from build123d import *

# Parameters (mm, degrees)
SKETCH_1_W          = 18
SKETCH_1_H          = 49
EXTRUDE_1_DEPTH     = 2
CUT_EXTRUDE_1_DEPTH = 0.1


with BuildPart() as part:
    # ｽｹｯﾁ1 → ﾎﾞｽ - 押し出し1 (new body)
    with BuildSketch(Plane.XY):
        with Locations((9, 24.5)):
            Rectangle(SKETCH_1_W, SKETCH_1_H)
    extrude(amount=EXTRUDE_1_DEPTH)

    # ｽｹｯﾁ2 → ｶｯﾄ - 押し出し1 (cut)
    with BuildSketch(Plane.XY.offset(2)):
        with BuildLine():
            add(Edge.make_bspline(
                [(0.915865385, 24.396709736), (0.91809708, 24.77837232), (0.922432179, 25.519757391), (0.970658757, 26.600060045), (1.05077314, 27.613522012), (1.160564909, 28.5601918), (1.29417331, 29.440313805), (1.472532246, 30.251535992), (1.675365778, 30.997612959), (1.910445811, 31.68097761), (2.175702018, 32.310836625), (2.464406542, 32.898836655), (2.788017018, 33.444088016), (3.128038515, 33.95529334), (3.498234931, 34.42408455), (3.888071345, 34.85708195), (4.312763039, 35.244278306), (4.757873149, 35.597018327), (5.227431594, 35.906237054), (5.708054019, 36.178602651), (6.203048578, 36.411283891), (6.713766716, 36.594234892), (7.235618047, 36.745347974), (7.77042684, 36.848687065), (8.31907612, 36.913708174), (8.689404274, 36.919924378), (8.877216046, 36.923076923)],
                knots=[0, 0, 0, 0, 1.646270934, 3.197905019, 4.663502075, 6.030701355, 7.308322542, 8.50163776, 9.611534131, 10.641858119, 11.616356847, 12.558055219, 13.465016945, 14.349605745, 15.204443733, 16.039544428, 16.859896111, 17.680448484, 18.487036065, 19.28249412, 20.06191084, 20.843045899, 21.620316918, 22.403196591, 23.190181807, 24, 24, 24, 24], degree=3))
            add(Edge.make_bspline(
                [(8.877216046, 36.923076923), (9.066596712, 36.919758038), (9.443215272, 36.913157819), (10.000022111, 36.84972171), (10.543965481, 36.744462819), (11.072726389, 36.595321902), (11.590648172, 36.410294174), (12.093679803, 36.178380038), (12.58494584, 35.908422029), (13.056639404, 35.59121315), (13.51393884, 35.237548021), (13.945611588, 34.837752006), (14.351696941, 34.395861952), (14.737291429, 33.916605699), (15.091455403, 33.390791104), (15.42873179, 32.8275635), (15.730620106, 32.217073152), (16.021368521, 31.569506041), (16.27233177, 30.866944362), (16.498661046, 30.113348402), (16.681534028, 29.299816881), (16.833861042, 28.43061814), (16.95186828, 27.502560085), (17.037815363, 26.517632117), (17.083216174, 25.475186245), (17.09176623, 24.762458735), (17.096153846, 24.396709736)],
                knots=[0, 0, 0, 0, 0.810914788, 1.612654377, 2.396697861, 3.181598691, 3.963628158, 4.749916497, 5.551656086, 6.361998678, 7.18212741, 8.025565596, 8.878627764, 9.750805457, 10.657531673, 11.591944965, 12.560506719, 13.57287815, 14.630710178, 15.753379473, 16.941251878, 18.199788006, 19.531962791, 20.947069417, 22.433333509, 24, 24, 24, 24], degree=3))
            add(Edge.make_bspline(
                [(17.096153846, 24.396709736), (17.091720744, 24.032556005), (17.083083026, 23.323017311), (17.038324324, 22.285261925), (16.950159351, 21.305560952), (16.839873538, 20.38156477), (16.687126808, 19.517119185), (16.499313088, 18.709232848), (16.290781427, 17.954416932), (16.033369703, 17.258855088), (15.751628977, 16.61284426), (15.445092732, 16.009590983), (15.116685522, 15.44376317), (14.758894239, 14.919889892), (14.377530838, 14.4342601), (13.964433025, 13.995445917), (13.531245652, 13.592874024), (13.072600465, 13.234654916), (12.593550447, 12.921113656), (12.103971728, 12.640712281), (11.595177637, 12.414611266), (11.078698441, 12.220471077), (10.547146522, 12.072150145), (10.001184471, 11.969594092), (9.443589365, 11.897667766), (9.06666086, 11.892180823), (8.877216046, 11.889423077)],
                knots=[0, 0, 0, 0, 1.561518951, 3.042555995, 4.452378317, 5.7783523, 7.031515105, 8.214008947, 9.334062868, 10.386615937, 11.391082383, 12.354592575, 13.286541444, 14.194233754, 15.072674879, 15.931287219, 16.775624067, 17.606195743, 18.42308326, 19.229000347, 20.022332153, 20.807536673, 21.593273796, 22.3848459, 23.188221202, 24, 24, 24, 24], degree=3))
            add(Edge.make_bspline(
                [(8.877216046, 11.889423077), (8.689409484, 11.89259596), (8.319091603, 11.898852265), (7.770367066, 11.963579617), (7.237766871, 12.067643665), (6.718662848, 12.213353061), (6.210391736, 12.391707572), (5.7198795, 12.624074598), (5.241672223, 12.891686746), (4.777045744, 13.196455595), (4.334730863, 13.545626332), (3.912238566, 13.931826225), (3.520182632, 14.364692648), (3.155279232, 14.837390661), (2.808473382, 15.34557147), (2.489458181, 15.896173437), (2.194381478, 16.487013341), (1.924664157, 17.121908411), (1.685527714, 17.810123188), (1.474292414, 18.559530992), (1.307508593, 19.376746302), (1.164749558, 20.255205532), (1.049603309, 21.198683523), (0.970992631, 22.207692478), (0.922406184, 23.281603631), (0.918085437, 24.018224774), (0.915865385, 24.396709736)],
                knots=[0, 0, 0, 0, 0.810891512, 1.598919785, 2.382837074, 3.152667961, 3.926044502, 4.706494248, 5.493654104, 6.291793342, 7.103789334, 7.925228297, 8.761435821, 9.622817696, 10.50288917, 11.416980706, 12.369136599, 13.353924996, 14.394355917, 15.514179734, 16.714354668, 17.994756427, 19.357759367, 20.818452758, 22.365282078, 24, 24, 24, 24], degree=3))
        make_face()
        with BuildLine():
            add(Edge.make_bspline(
                [(3.052884615, 24.40625), (3.053697282, 24.088191888), (3.055274508, 23.470903548), (3.096478302, 22.573898505), (3.152609344, 21.737261089), (3.22500817, 20.959928993), (3.332524659, 20.244533372), (3.452994055, 19.586153921), (3.599598021, 18.988274861), (3.773055197, 18.446793506), (3.970624767, 17.95252038), (4.186337875, 17.492590684), (4.418072436, 17.061571259), (4.6774188, 16.663333674), (4.959869498, 16.296579236), (5.259044707, 15.954816573), (5.586109968, 15.650037111), (6.03857293, 15.284502615), (6.635902515, 14.906774223), (7.388516684, 14.577848147), (8.161868109, 14.371138935), (8.68677215, 14.344851595), (8.948768029, 14.331730769)],
                knots=[0, 0, 0, 0, 1.459021318, 2.831673884, 4.118529203, 5.306027144, 6.411944654, 7.436330062, 8.375795394, 9.233974572, 10.042671642, 10.816086306, 11.563610507, 12.285937304, 12.993564865, 13.685989202, 14.367179055, 15.041617293, 16.353048772, 17.594441528, 18.799311195, 20, 20, 20, 20], degree=3))
            add(Edge.make_bspline(
                [(8.948768029, 14.331730769), (9.212458616, 14.342601385), (9.739295369, 14.364320173), (10.509009225, 14.573861583), (11.256247313, 14.890020414), (11.841843906, 15.263859692), (12.287359068, 15.619879219), (12.606562162, 15.923418165), (12.899537884, 16.263296477), (13.177409858, 16.630004187), (13.432265355, 17.030547338), (13.664016345, 17.462999859), (13.87549412, 17.928562659), (13.995978879, 18.253567491), (14.057579627, 18.419734075)],
                knots=[0, 0, 0, 0, 1.353760809, 2.704726607, 4.075137775, 5.516104923, 6.260822281, 7.007110065, 7.778089737, 8.566572457, 9.372053459, 10.217411131, 11.088608312, 12, 12, 12, 12], degree=3))
            add(Edge.make_bspline(
                [(14.057579627, 18.419734075), (14.129369333, 18.632207838), (14.275133224, 19.063620698), (14.462991902, 19.732844831), (14.610938279, 20.434992207), (14.744039035, 21.165866662), (14.834887505, 21.930858199), (14.90801102, 22.727599847), (14.951082301, 23.556692329), (14.956421411, 24.119993966), (14.959134615, 24.40625)],
                knots=[0, 0, 0, 0, 0.884706709, 1.796334032, 2.740027952, 3.714592787, 4.726048262, 5.777819803, 6.87074269, 8, 8, 8, 8], degree=3))
            add(Edge.make_bspline(
                [(14.959134615, 24.40625), (14.955391364, 24.692459734), (14.948068763, 25.252347159), (14.920078954, 26.07230121), (14.847800706, 26.851090797), (14.767524558, 27.592070977), (14.649161322, 28.291140001), (14.521541243, 28.954150114), (14.350082995, 29.572887479), (14.166932383, 30.157039276), (13.957311656, 30.699968729), (13.726563536, 31.204207168), (13.480126213, 31.672188956), (13.212458469, 32.102630112), (12.92673784, 32.497458663), (12.615423086, 32.848758316), (12.290862978, 33.167416974), (11.836267481, 33.531153381), (11.241129902, 33.902027595), (10.500590766, 34.243333926), (9.729945847, 34.439333202), (9.208972883, 34.46696718), (8.948768029, 34.480769231)],
                knots=[0, 0, 0, 0, 1.31362396, 2.569729283, 3.763502607, 4.902122613, 5.988968491, 7.01645872, 7.998833611, 8.933434873, 9.825090667, 10.667526885, 11.477055099, 12.250526234, 12.991942729, 13.710640831, 14.402115721, 15.076753259, 16.378508321, 17.609869233, 18.806226677, 20, 20, 20, 20], degree=3))
            add(Edge.make_bspline(
                [(8.948768029, 34.480769231), (8.685397751, 34.466948138), (8.158177396, 34.439280775), (7.379522561, 34.244064175), (6.633141169, 33.903797389), (6.039577359, 33.529924997), (5.584664812, 33.173837557), (5.264334344, 32.865047575), (4.963982708, 32.527275737), (4.687297106, 32.157148424), (4.428153947, 31.759375121), (4.190158129, 31.330826561), (3.975727725, 30.869331029), (3.777849006, 30.375279924), (3.603862716, 29.833845284), (3.46034843, 29.236702667), (3.327766873, 28.580417296), (3.233909775, 27.861147072), (3.150472437, 27.083620279), (3.096851123, 26.244894239), (3.055136675, 25.346384794), (3.053650337, 24.725904805), (3.052884615, 24.40625)],
                knots=[0, 0, 0, 0, 1.207732386, 2.417664972, 3.655092373, 4.956220595, 5.625982001, 6.301752483, 6.994047911, 7.697131622, 8.419323945, 9.170223765, 9.943494443, 10.752040957, 11.610060368, 12.549350801, 13.567764191, 14.679664412, 15.874934091, 17.154273443, 18.533957287, 20, 20, 20, 20], degree=3))
        make_face(mode=Mode.SUBTRACT)
    extrude(amount=-CUT_EXTRUDE_1_DEPTH, mode=Mode.SUBTRACT)


solid = part.part
Design review of the part built by this model. Coordinates are the model's own, in mm. Coordinates: 2 decimals unless noted, no trailing zeros. Use one line per item in the form item = value.
(1) Draft analysis for pull direction X (two halves, no side actions). For faces 1 (the face through (2, 25, 1.9)), 2 (the face through (0, 24, 1)), 3 (the face through (9, 49, 1)), state which applies: pulls with the +X half, pulls with the -X half, needs draft (parallel to the pull), parting line crosses it, or undercut.
Return value:
face_1 = undercut
face_2 = pulls with the -X half
face_3 = needs draft
(2) For line 1 along Z through (x, y) = (1, 24.5), list the stretches that pass through material, from the lowest coordinate up. Write a range as from..to.
Return value:
line_1 = 0..1.9
(3) Clearance check with a flat-ended pin moving along its axis: P1, Ø2, axis at x = 15.5, y = 21.5, coming from the +Z side. State where the tip first meets the part, or that it passes through.
Return value:
P1 = 2
